Job drawing, mm, ordinate dimensions from the low corner. One solid piece. Give positions to 0.01 mm unless a question says otherwise; leave off trailing zeros. Loops run counter-clockwise (first coordinate to the right, second up) from the corner with the lowest first, then second, coordinate; pieces in that order, holes last.
Item 1: Probe probe 1 along Y at (x, z) = (20, 1.5); probe 2 along X at (y, z) = (59.5, 0.6); probe 3 along Y at (x, z) = (24, 1.8). List the from-to ranges inside material, lowest first.
Item 2: Saw through at C-C on z = 0.75. Give the cut face in (x, y).
Item 3: Drop a flat-ended pin along its axis: P1, Ø7, axis at x = 20, y = 20, coming from the -Z side. Give the stop position or say it passes through.
Item 4: Saw through at A-A on y = 60. Give the cut face in (x, z), plus the area to 3 significant figures.
Item 5: Saw through at B-B on x = 60. Give the cut face in (y, z), plus the area to 3 significant figures.
Item 6: Saw through at D-D on y = 98. Give the cut face in (x, z).
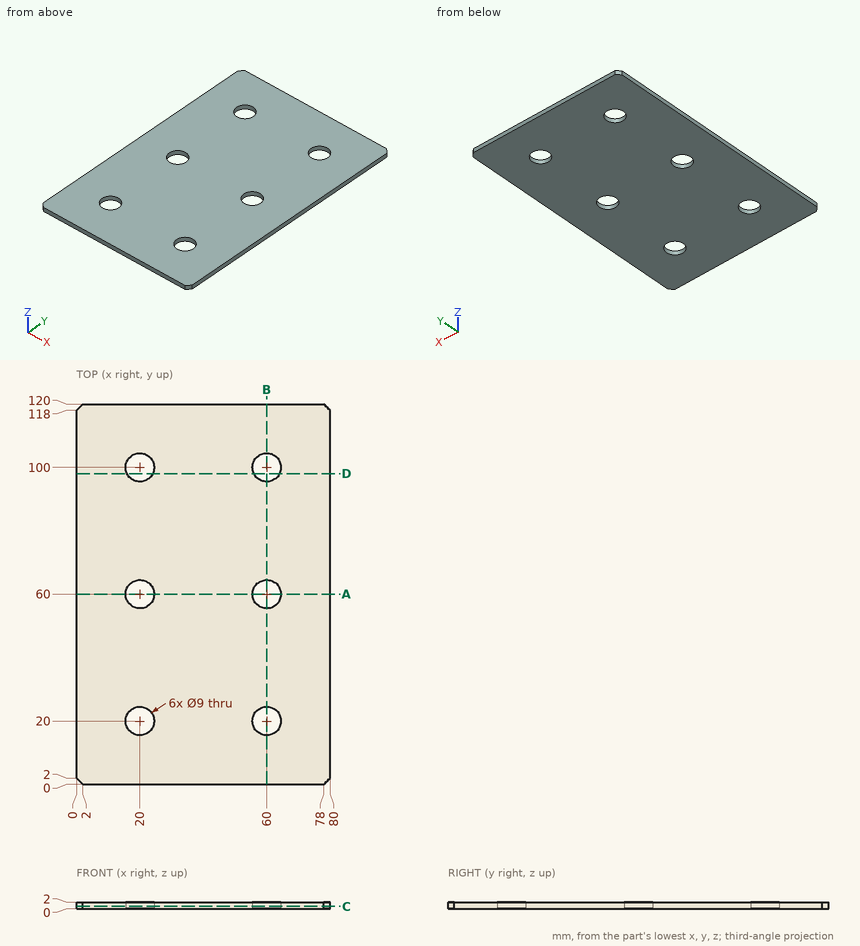
Results below:
1. probe 1: y = 0 to 15.5, 24.5 to 55.5, 64.5 to 95.5, 104.5 to 120
1. probe 2: x = 0 to 15.53, 24.47 to 55.53, 64.47 to 80
1. probe 3: y = 0 to 17.94, 22.06 to 57.94, 62.06 to 97.94, 102.06 to 120
2. outline: (0, 2) - (2, 0) - (78, 0) - (80, 2) - (80, 118) - (78, 120) - (2, 120) - (0, 118) - close; hole circle Ø9 at (20, 20); hole circle Ø9 at (20, 60); hole circle Ø9 at (20, 100); hole circle Ø9 at (60, 20); hole circle Ø9 at (60, 60); hole circle Ø9 at (60, 100)
3. P1: passes through
4. outline: (0, 0) - (15.5, 0) - (15.5, 2) - (0, 2) - close; (24.5, 0) - (55.5, 0) - (55.5, 2) - (24.5, 2) - close; (64.5, 0) - (80, 0) - (80, 2) - (64.5, 2) - close
4. area: 124 mm2
5. outline: (0, 0) - (15.5, 0) - (15.5, 2) - (0, 2) - close; (24.5, 0) - (55.5, 0) - (55.5, 2) - (24.5, 2) - close; (64.5, 0) - (95.5, 0) - (95.5, 2) - (64.5, 2) - close; (104.5, 0) - (120, 0) - (120, 2) - (104.5, 2) - close
5. area: 186 mm2
6. outline: (0, 0) - (15.97, 0) - (15.97, 2) - (0, 2) - close; (24.03, 0) - (55.97, 0) - (55.97, 2) - (24.03, 2) - close; (64.03, 0) - (80, 0) - (80, 2) - (64.03, 2) - close
